from build123d import *

# Parameters (mm, degrees)
F0_W      = 60
F0_H      = 50
F0_R      = 5.5
F1_DEPTH  = 2
F2_W      = 40
F2_H      = 25
F2_R      = 5.5
F3_DEPTH  = 10
F4_R      = 10
F5_W      = 60
F5_H      = 50
F5_R      = 5.5
F6_DEPTH  = 2
F7_R      = 4
F9_D      = 1
F9_DEPTH  = 3
F9_TIP    = 0.3004303095
F10_W     = 7.5
F10_H     = 17
F11_DEPTH = 25
F12_R     = 5


# Not quite as in the source:
# - a feature names something its author has since deleted; it is built from what else it names


with BuildPart() as f1:
    # F0 (on Front) → F1 (new body)
    with BuildSketch(Plane.XZ):
        with Locations((0, 2.5)):
            Rectangle(F0_W, F0_H)
        Circle(F0_R, mode=Mode.SUBTRACT)
    extrude(amount=F1_DEPTH)

    # F2 (on face) → F3 (join)
    with BuildSketch(Plane.XZ.offset(2)):
        Rectangle(F2_W, F2_H)
        Circle(F2_R, mode=Mode.SUBTRACT)
    extrude(amount=F3_DEPTH)

    # F4
    f4_edges = [f1.edges().sort_by_distance(p)[0] for p in [
        (20, -7, 12.5),
        (20, -7, -12.5),
        (-20, -7, -12.5),
        (-20, -7, 12.5),
    ]]
    fillet(f4_edges, radius=F4_R)

    # F5 (on face) → F6 (join)
    with BuildSketch(Plane.XZ.offset(12)):
        with Locations((0, 2.5)):
            Rectangle(F5_W, F5_H)
        Circle(F5_R, mode=Mode.SUBTRACT)
    extrude(amount=F6_DEPTH)

    # F7
    f7_edges = [f1.edges().sort_by_distance(p)[0] for p in [
        (30, -13, 27.5),
        (30, -1, 27.5),
        (30, -13, -22.5),
        (30, -1, -22.5),
        (-30, -13, -22.5),
        (-30, -1, -22.5),
        (-30, -13, 27.5),
        (-30, -1, 27.5),
    ]]
    fillet(f7_edges, radius=F7_R)

    # F9
    with Locations(Plane.XZ.offset(14)):
        with Locations((-19, 10.5), (-27, -19.5), (27, -19.5)):
            Hole(F9_D / 2, depth=F9_DEPTH)
            with Locations((0, 0, -(F9_DEPTH + F9_TIP / 2))):  # 118° drill point
                Cone(0, F9_D / 2, F9_TIP, mode=Mode.SUBTRACT)

    # F10 (on face) → F11 (cut)
    with BuildSketch(Plane.XZ.offset(14)):
        with Locations((-12.25, 0)):
            Rectangle(F10_W, F10_H)
        with Locations((12.25, 0)):
            Rectangle(F10_W, F10_H)
    extrude(amount=-F11_DEPTH, mode=Mode.SUBTRACT)

    # F12
    f12_edges = [f1.edges().sort_by_distance(p)[0] for p in [
        (16, -7, -8.5),
        (16, -7, 8.5),
        (-16, -7, 8.5),
        (-16, -7, -8.5),
    ]]
    fillet(f12_edges, radius=F12_R)


solid = f1.part
Check sheet for the modelled part. Datum: model origin and axes. Units: mm. A direction names the side the tool comes from. Give positions to 0.01 mm unless a question says otherwise; leave off trailing zeros. Write each loop counter-clockwise with the first axis right and the second up, starting at its lowest first coordinate (ties: lowest second). Pieces come first, ordered by that corner, then holes. Notation, with made-up numbers: (52, 40.25) -> (90, 40.25) arc R18 cw to (90, 44.25) -> close; hole circle Ø5 at (73.25, 44). An arc over 180 degrees is marked (long way). Write item = value, one per line.
Item 1: Release check for a two-part mould opening along Z. For faces 6 (the flat face through (30, -1, 2)), 7 (the flat face through (0, -7, -12.5)), 8 (the flat face through (10, -7, -8.5)), 9 (the flat face through (-8.5, -7, 0)) record: +Z half, -Z half, draft (parallel to the pull), parting line (faces both ways), or undercut.
Output:
face_6 = draft
face_7 = -Z half
face_8 = undercut
face_9 = undercut
Item 2: Tool access check on faces 1 (the cylindrical face through (17.15, -7.07, -9.49)), 2 (the cylindrical face through (17.15, -7.07, 9.49)), 3 (the cylindrical face through (-28.797, -1.014, 26.359)), 4 (the flat face through (-20, -7, 0)), 5 (the flat face through (-16, -7, 0)). Record the directions out of +Z, -Z, +X, -X, +Y, -Y that give a thin tool (end or side, any length) a straight path to the whole face; none if there is none.
Output:
face_1 = -Z, +X
face_2 = +Z, +X
face_3 = +Z, -X, +Y, -Y
face_4 = +Z, -Z, -X
face_5 = +Y, -Y
Item 3: Sectioned sample at A-A on x = -23.5. Record the boundary of the cut face in (y, z), and give its area (3 significant figures).
Output:
outline = (-14, -22.5) -> (-12, -22.5) -> (-12, 27.5) -> (-14, 27.5) -> close; (-2, -22.5) -> (0, -22.5) -> (0, 27.5) -> (-2, 27.5) -> close
area = 200 mm^2
Item 4: Sectioned sample at C-C on z = 20. Record the boundary of the cut face in (x, y).
Output:
outline = (-30, -14) -> (30, -14) -> (30, -12) -> (-30, -12) -> close; (-30, -2) -> (30, -2) -> (30, 0) -> (-30, 0) -> close
Item 5: Sectioned sample at B-B on y = -12.75. Record the boundary of the cut face in (x, z), and give its area (3 significant figures).
Output:
outline = (-30, -18.5) arc R4 ccw to (-26, -22.5) -> (26, -22.5) arc R4 ccw to (30, -18.5) -> (30, 23.5) arc R4 ccw to (26, 27.5) -> (-26, 27.5) arc R4 ccw to (-30, 23.5) -> close; hole circle Ø1 at (-27, -19.5); hole circle Ø1 at (-19, 10.5); hole (-16, -3.5) arc R5 ccw to (-11, -8.5) -> (-8.5, -8.5) -> (-8.5, 8.5) -> (-11, 8.5) arc R5 ccw to (-16, 3.5) -> close; hole circle Ø11 at (0, 0); hole (8.5, -8.5) -> (11, -8.5) arc R5 ccw to (16, -3.5) -> (16, 3.5) arc R5 ccw to (11, 8.5) -> (8.5, 8.5) -> close; hole circle Ø1 at (27, -19.5)
area = 2,660 mm^2
Item 6: Gauge pin test, flat ends, axial feed: pin 1 (5.5 mm diameter, centred on y = -8.5, z = -1.5, fed in from -X); pin 2 (0.8 mm diameter, centred on x = -9.5, y = -10, fed in from +Z); pin 3 (2 mm diameter, centred on y = -9.5, z = -0.5, fed in from +X). Record the tip position at first contact, or that the pin passes through.
Output:
pin_1 = -20
pin_2 = 12.5
pin_3 = 20
Item 7: Sectioned sample at D-D on z = 0. Record the boundary of the cut face in (x, y).
Output:
outline = (-30, -14) -> (-16, -14) -> (-16, 0) -> (-30, 0) -> (-30, -2) -> (-20, -2) -> (-20, -12) -> (-30, -12) -> close; (-8.5, -14) -> (-5.5, -14) -> (-5.5, 0) -> (-8.5, 0) -> close; (5.5, -14) -> (8.5, -14) -> (8.5, 0) -> (5.5, 0) -> close; (16, -14) -> (30, -14) -> (30, -12) -> (20, -12) -> (20, -2) -> (30, -2) -> (30, 0) -> (16, 0) -> close
Item 8: Scan lines: probe 1 along Y at (x, z) = (27, 0.5); probe 2 along Z at (x, y) = (0, -6.25); probe 3 along X at (y, z) = (-2.5, 4). Record each from-to range of solid material in increasing order. Write a range as from..to.
Output:
probe_1 = -14..-12, -2..0
probe_2 = -12.5..-5.5, 5.5..12.5
probe_3 = -19.89..-15.97, -8.5..-3.77, 3.77..8.5, 15.97..19.89
